from build123d import *

# Parameters (mm, degrees)
FLEXURE_BOSS_DEPTH            = 4.18
SKETCH2_W                     = 9.5
SKETCH2_H                     = 18
SKETCH2_R                     = 1.575
MOUNTING_PLATE_BOSS_DEPTH     = 1
DOVETAIL_CONNECTION_CUT_DEPTH = 3.68


with BuildPart() as part:
    # Sketch1 → Flexure Boss (new body)
    with BuildSketch(Plane(origin=(0, 0, 0), x_dir=(0, 0, -1), z_dir=(1, 0, 0))):
        with BuildLine():
            Line((2.368651747, -1.066915143), (8.368651984, -1.066915143))
            Line((8.368651984, -1.066915143), (8.368651984, 5.083084857))
            Line((8.368651984, 5.083084857), (-4.631348016, 5.083084857))
            Line((-4.631348016, 5.083084857), (-4.631348016, -1.066915143))
            Line((-4.631348016, -1.066915143), (-1.631348253, -1.066915143))
            ThreePointArc((-1.631348253, -1.066915143), (-0.924241471, -1.359808362), (-0.631348253, -2.066915143))
            Line((-0.631348253, -2.066915143), (-0.631348253, -11.066916497))
            Line((-0.631348253, -11.066916497), (6.427805299, -11.066916497))
            Line((6.427805299, -11.066916497), (6.427805299, -11.816916497))
            Line((6.427805299, -11.816916497), (-0.63134937, -11.816916497))
            ThreePointArc((-0.63134937, -11.816916497), (-1.338456151, -11.524023278), (-1.63134937, -10.816916497))
            Line((-1.63134937, -10.816916497), (-1.63134937, -1.566915143))
            Line((-1.63134937, -1.566915143), (-3.63134937, -1.566915143))
            Line((-3.63134937, -1.566915143), (-3.63134937, -13.316915143))
            Line((-3.63134937, -13.316915143), (-4.631348016, -13.316915143))
            Line((-4.631348016, -13.316915143), (-4.631348016, -14.816915143))
            Line((-4.631348016, -14.816915143), (17.924748705, -14.816915143))
            Line((17.924748705, -14.816915143), (16.743651747, -1.316915143))
            Line((16.743651747, -1.316915143), (14.743651747, -1.316915143))
            Line((14.743651747, -1.316915143), (14.743651747, -11.816915143))
            Line((14.743651747, -11.816915143), (13.993651747, -11.816915143))
            Line((13.993651747, -11.816915143), (13.993651747, -1.316915143))
            Line((13.993651747, -1.316915143), (11.993651747, -1.316915143))
            Line((11.993651747, -1.316915143), (11.993651747, -11.816915143))
            Line((11.993651747, -11.816915143), (11.243651747, -11.816915143))
            Line((11.243651747, -11.816915143), (11.243651747, -1.816915143))
            Line((11.243651747, -1.816915143), (8.743651747, -1.816915143))
            Line((8.743651747, -1.816915143), (8.743651747, -2.316915143))
            Line((8.743651747, -2.316915143), (1.868651747, -2.316915143))
            Line((1.868651747, -2.316915143), (1.868651747, -4.066915143))
            Line((1.868651747, -4.066915143), (8.743651747, -4.066915143))
            Line((8.743651747, -4.066915143), (8.743651747, -4.566915143))
            ThreePointArc((8.743651747, -4.566915143), (8.670428443, -4.743691838), (8.493651747, -4.816915143))
            Line((8.493651747, -4.816915143), (1.368651747, -4.816915143))
            Line((1.368651747, -4.816915143), (1.368651747, -2.066915143))
            ThreePointArc((1.368651747, -2.066915143), (1.661544966, -1.359808362), (2.368651747, -1.066915143))
        make_face()
        with BuildLine():
            Line((0.493651747, -9.816916497), (9.618651747, -9.816916497))
            Line((9.618651747, -9.816916497), (9.618651747, -3.566915143))
            Line((9.618651747, -3.566915143), (2.868650393, -3.566915143))
            Line((2.868650393, -3.566915143), (2.868650393, -2.816915143))
            Line((2.868650393, -2.816915143), (9.618651747, -2.816915143))
            ThreePointArc((9.618651747, -2.816915143), (10.325758529, -3.109808362), (10.618651747, -3.816915143))
            Line((10.618651747, -3.816915143), (10.618651747, -12.816913789))
            Line((10.618651747, -12.816913789), (12.618651747, -12.816913789))
            Line((12.618651747, -12.816913789), (12.618651747, -2.316912435))
            Line((12.618651747, -2.316912435), (13.368651747, -2.316912435))
            Line((13.368651747, -2.316912435), (13.368651747, -12.816913789))
            Line((13.368651747, -12.816913789), (15.368651747, -12.816913789))
            Line((15.368651747, -12.816913789), (15.368651747, -2.316912435))
            Line((15.368651747, -2.316912435), (16.118651747, -2.316912435))
            Line((16.118651747, -2.316912435), (17.081027283, -13.316915143))
            Line((17.081027283, -13.316915143), (-3.00634937, -13.316915143))
            Line((-3.00634937, -13.316915143), (-3.00634937, -2.566915143))
            Line((-3.00634937, -2.566915143), (-2.25634937, -2.566915143))
            Line((-2.25634937, -2.566915143), (-2.25634937, -12.816916497))
            Line((-2.25634937, -12.816916497), (0.24365063, -12.816916497))
            Line((0.24365063, -12.816916497), (0.24365063, -12.316916497))
            Line((0.24365063, -12.316916497), (7.11865063, -12.316916497))
            Line((7.11865063, -12.316916497), (7.11865063, -10.566916497))
            Line((7.11865063, -10.566916497), (0.243651747, -10.566916497))
            Line((0.243651747, -10.566916497), (0.243651747, -10.066916497))
            ThreePointArc((0.243651747, -10.066916497), (0.316875052, -9.890139802), (0.493651747, -9.816916497))
        make_face(mode=Mode.SUBTRACT)
    extrude(amount=FLEXURE_BOSS_DEPTH)

    # Sketch2 → Mounting Plate Boss (add)
    with BuildSketch(Plane.XZ.offset(14.816915143)):
        with Locations((-0.57, -16.309568548)):
            Rectangle(SKETCH2_W, SKETCH2_H)
        with Locations(Location((-1.75, -10.088651984, 0), (0, 0, 270))):
            Circle(SKETCH2_R, mode=Mode.SUBTRACT)
        with Locations(Location((-1.75, -22.088651984, 0), (0, 0, 270))):
            Circle(SKETCH2_R, mode=Mode.SUBTRACT)
    extrude(amount=-MOUNTING_PLATE_BOSS_DEPTH)

    # Sketch7 → Dovetail Connection Cut (cut)
    with BuildSketch(Plane.ZY):
        Polygon((-8.368651984, 0.933084857), (4.631348016, 0.933084857), (4.631348016, 4.083084857), (-1.868651984, 3.083084857), (-8.368651984, 4.083084857), align=None)
    extrude(amount=-DOVETAIL_CONNECTION_CUT_DEPTH, mode=Mode.SUBTRACT)


solid = part.part
Geometry check sheet. Reference: the model listing, model coordinates, mm. A direction names the side the tool comes from. Give positions to 0.01 mm unless a question says otherwise; leave off trailing zeros. Loops run counter-clockwise (first coordinate to the right, second up) from the corner with the lowest first, then second, coordinate; pieces in that order, holes last. Notation, with made-up numbers: M 16,66.5 L 60,66.5 A20 ccw 60,96.5 Z; hole C 36,40.25 d5. An arc over 180 degrees is marked long. Write each question's results on one line, items separated by ' | '.
1) Gauge pin test, flat ends, axial feed: pin 1 (8 mm diameter, centred on y = -7.5, z = 0.5, fed in from -X); pin 2 (4 mm diameter, centred on x = -1.5, z = -0.5, fed in from +Y); pin 3 (1.3 mm diameter, centred on x = 2.5, y = -7.5, fed in from -Z); pin 4 (0.6 mm diameter, centred on x = 2.5, y = -3, fed in from -Z). Record the tip position at first contact, or that the pin passes through.
Answers follow:
pin 1: x = 0 | pin 2: y = 5.08 | pin 3: z = -17.34 | pin 4: z = -16.92
2) Release check for a two-part mould opening along Z. For faces 4 (the face through (2.1, 0.6, -8.369)), 5 (the face through (-2.71, -14.32, -20.84)), 6 (the face through (-5.32, -14, -16)) record: +Z half, -Z half, draft (parallel to the pull), parting line (faces both ways), or undercut.
Answers follow:
face 4: -Z half | face 5: undercut | face 6: draft
3) Tool access check on faces 1 (the face through (2, -6, -11.994)), 2 (the face through (2, -6, 1.631)), 3 (the face through (2, -1.067, -5)). Record the directions out of +Z, -Z, +X, -X, +Y, -Y that give a thin tool (end or side, any length) a straight path to the whole face; none if there is none.
Answers follow:
face 1: +X, -X, +Y | face 2: +X, -X | face 3: -Z, +X, -X
4) Section check B-B, the plane y = -6.5. Count the separate pieces of the cut face and the enclosed holes in it, plus the area to 3 significant figures.
Answers follow:
separate pieces: 8 | enclosed holes: 0 | area: 61.5 mm2
5) Section check A-A, the plane x = -1.75. Record the boundary of the cut face in (y, z).
Answers follow:
outline: M -14.82,-25.31 L -13.82,-25.31 L -13.82,-23.66 L -14.82,-23.66 Z; M -14.82,-20.51 L -13.82,-20.51 L -13.82,-11.66 L -14.82,-11.66 Z; M -14.82,-8.51 L -13.82,-8.51 L -13.82,-7.31 L -14.82,-7.31 Z
6) Thickness scan on line 1 (Y direction, x = 0.5, z = -9.25); line 2 (Y direction, x = 2, z = 1); line 3 (Z direction, x = 0.5, y = -12). Record the ranges inside material, lowest first.
Answers follow:
line 1: -14.82 to -13.32, -9.82 to -3.57, -2.82 to -1.82 | line 2: -14.82 to -13.32, -12.82 to -11.75, -1.29 to 0.93, 3.52 to 5.08 | line 3: -17.68 to -16.97, -15.37 to -13.37, -12.62 to -10.62, -7.12 to 2.26, 3.01 to 3.63
7) Section check C-C, the plane z = -6.75. Record the boundary of the cut face in (x, y), plus the area to 3 significant figures.
Answers follow:
outline: M 0,-14.82 L 4.18,-14.82 L 4.18,-13.32 L 0,-13.32 Z; M 0,-12.32 L 4.18,-12.32 L 4.18,-10.57 L 0,-10.57 Z; M 0,-9.82 L 4.18,-9.82 L 4.18,-4.82 L 0,-4.82 Z; M 0,-4.07 L 4.18,-4.07 L 4.18,-3.57 L 0,-3.57 Z; M 0,-2.82 L 4.18,-2.82 L 4.18,-2.32 L 0,-2.32 Z; M 0,-1.07 L 4.18,-1.07 L 4.18,5.08 L 0,5.08 L 0,3.83 L 3.68,3.83 L 3.68,0.93 L 0,0.93 Z | area: 53.7 mm2
8) Section check D-D, the plane z = -21.5. Record the boundary of the cut face in (x, y).
Answers follow:
outline: M -5.32,-14.82 L -3.21,-14.82 L -3.21,-13.82 L -5.32,-13.82 Z; M -0.29,-14.82 L 4.18,-14.82 L 4.18,-13.82 L -0.29,-13.82 Z
